Check sheet for the drawn part. Datum: minimum x, y, z corner. Units: mm. A direction names the side the tool comes from. Give positions to 0.01 mm unless a question says otherwise; leave off trailing zeros. Write each loop counter-clockwise with the first axis right and the second up, starting at its lowest first coordinate (ties: lowest second). Pieces come first, ordered by that corner, then holes. Notation, with made-up numbers: (-20.5, -2) -> (-12.5, -2) arc R27 cw to (-12.5, 23) -> close; hole circle Ø2 at (31, -24). An arc over 180 degrees is marked (long way). Write item = value, one per line. Start each with the question number.
1. Depth check by flat-ended pin: P1, Ø0.9, axis at x = 27, z = 2, coming from the +Y side; P2, Ø1.5, axis at y = 26, z = 18, coming from the +X side; P3, Ø1, axis at x = 17, z = 9.5, coming from the +Y side; P4, Ø7, axis at x = 19, y = 19.5, coming from the -Z side. Enter the tip coordinate at first touch or a pass-through.
2. Mould release check, pull along Z, two halves, no side actions. Record for the marked faces 1, 2, 3 and 4: pulls with the +Z half, pulls with the -Z half, needs draft (parallel to the pull), parting line crosses it, or undercut.
3. Cross-section at A-A, the plane y = 23.5. Record the cut outline in (x, z), plus the area to 3 significant figures.
4. Set-up check for the marked faces 5, 6 and 7: record each of +Z, -Z, +X, -X, +Y, -Y from which the full face is reachable in a straight line by a thin tool's end or side.
5. Cross-section at D-D, the plane z = 6.75. Record the cut outline in (x, y), plus the area to 3 significant figures.
6. Thickness scan on line 1 along Z through (x, y) = (8.5, 15.25); line 2 along Y through (x, z) = (18.5, 6). Record the ranges inside material, lowest first.
7. Cross-section at C-C, the plane z = 17.75. Record the cut outline in (x, y).
8. Cross-section at B-B, the plane x = 25. Record the cut outline in (y, z), plus the area to 3 significant figures.
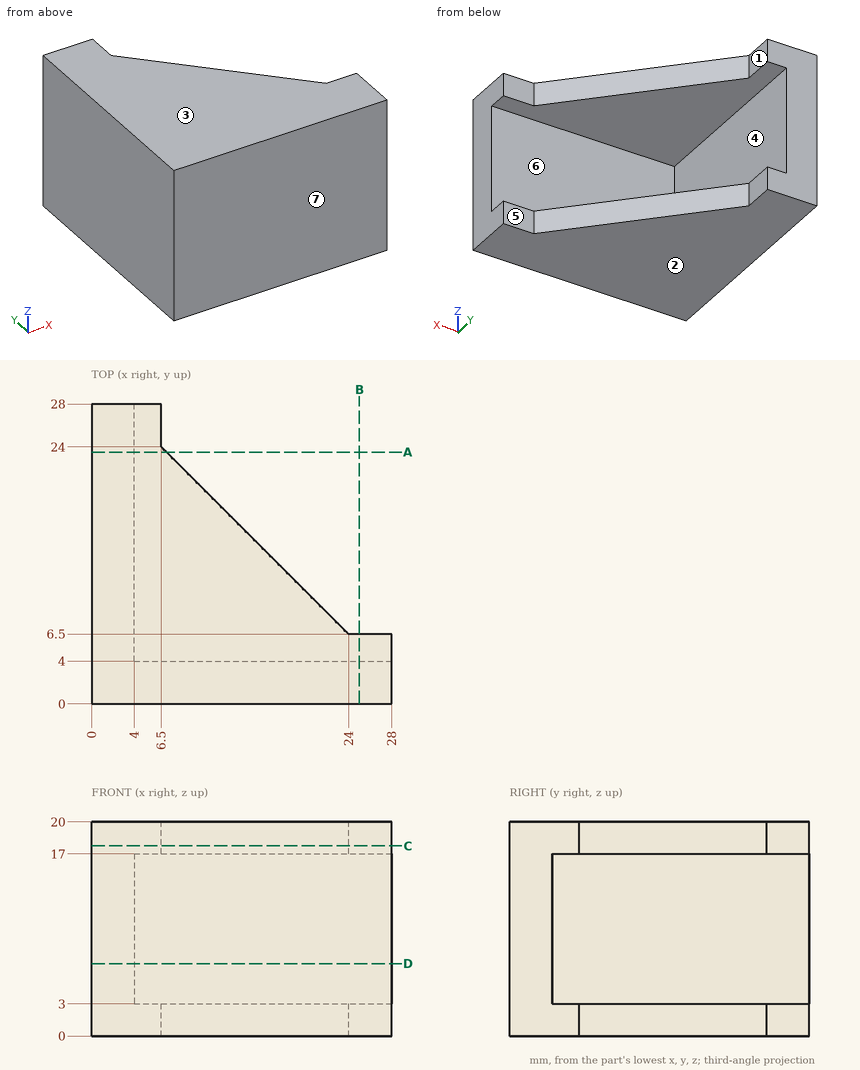
Answers:
q1.P1 = 6.5
q1.P2 = 6.5
q1.P3 = 4
q1.P4 = through
q2.face_1 = needs draft
q2.face_2 = pulls with the -Z half
q2.face_3 = pulls with the +Z half
q2.face_4 = undercut
q3.outline = (0, 0) -> (7, 0) -> (7, 3) -> (4, 3) -> (4, 17) -> (7, 17) -> (7, 20) -> (0, 20) -> close
q3.area = 98.0 mm^2
q4.face_5 = +Z, -Z, +X, +Y
q4.face_6 = +X, +Y
q4.face_7 = +Z, -Z, +X, -X, -Y
q5.outline = (0, 0) -> (28, 0) -> (28, 4) -> (4, 4) -> (4, 28) -> (0, 28) -> close
q5.area = 208 mm^2
q6.line_1 = 0 to 3, 17 to 20
q6.line_2 = 0 to 4
q7.outline = (0, 0) -> (28, 0) -> (28, 6.5) -> (24, 6.5) -> (6.5, 24) -> (6.5, 28) -> (0, 28) -> close
q8.outline = (0, 0) -> (6.5, 0) -> (6.5, 3) -> (4, 3) -> (4, 17) -> (6.5, 17) -> (6.5, 20) -> (0, 20) -> close
q8.area = 95.0 mm^2
